Can you work these out from the drawing? Everything is in mm from the part's minimum corner. A direction names the side the tool comes from. Round coordinates to 2 decimals unless told otherwise and drop trailing zeros. Write each loop counter-clockwise with the first axis right and the second up, starting at its lowest first coordinate (ties: lowest second). Pieces come first, ordered by that corner, then holes. Notation, with made-up numbers: (17.25, -27.75) -> (59.25, -27.75) arc R34 ccw to (59.25, 8.25) -> close; hole circle Ø4 at (57.5, 29). An arc over 180 degrees is marked (long way). Answer as CSV lines item,"result". Start each with the question number.
Q1. If I drill on line 1 (Y direction, x = 11.55, z = 17.5); line 2 (Y direction, x = 13.25, z = 17.5); line 3 (X direction, y = 15.5, z = 11.5), over which ranges is the centre line in solid material (lowest first)? Write a range as [from, to].
Q2. For the marked faces 1 and 2, which set-ups out of +Z, -Z, +X, -X, +Y, -Y let a thin tool reach every point of the face, with its end or its side?
Q3. Imagine slicing it at D-D on x = 8. Please give me the cut outline in (y, z).
Q4. If we mould it in two halves opening along Y, with no side actions, what happens to the marked faces 3, 4 and 5? For each: pulls with the +Y half, pulls with the -Y half, needs draft (parallel to the pull), parting line crosses it, or undercut.
Q5. Imagine slicing it at A-A on z = 17.5. Please give me the cut outline in (x, y), and give its area (3 significant figures).
Q6. Will these pins go through, and if not, where does the flat tip stop? pin 1 Ø3 at (y, z) = (46.5, 3.5) entering from +X; pin 2 Ø5 at (y, z) = (8.5, 17.5) entering from +X; pin 3 Ø6.5 at (x, y) = (9.5, 9.5) entering from +Z; pin 4 Ø10 at (x, z) = (8, 10.5) entering from +Y.
Q7. Imagine slicing it at B-B on y = 8. Please give me the cut outline in (x, z), and give its area (3 significant figures).
Q8. Imagine slicing it at C-C on z = 10.5. Please give me the cut outline in (x, y).
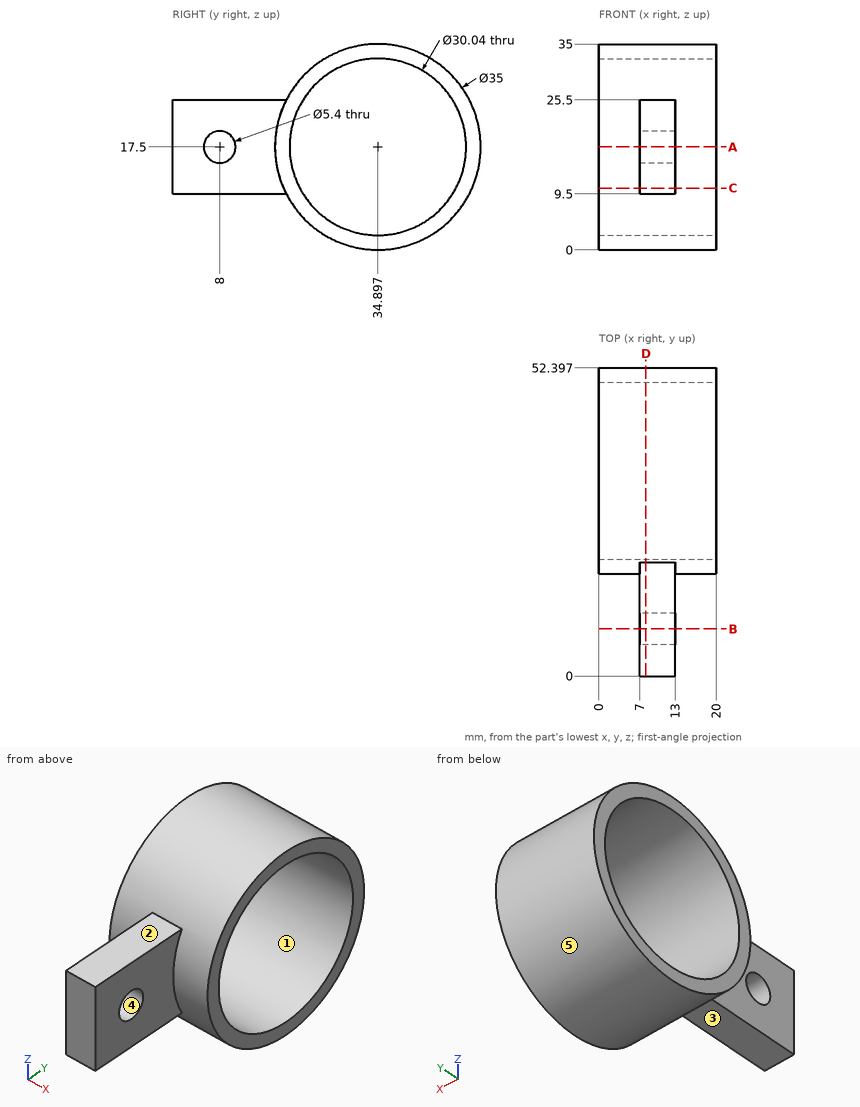
Checks:
1,line 1,"[0, 5.3], [10.7, 19.88], [49.92, 52.4]"
1,line 2,"[17.4, 19.88], [49.92, 52.4]"
1,line 3,"[7, 13]"
2,face 1,"+X, -X"
2,face 2,"+Z, +X, -X, -Y"
3,outline,"(0, 9.5) -> (19.33, 9.5) arc R17.5 ccw (long way) to (19.33, 25.5) -> (0, 25.5) -> close; hole circle Ø5.4 at (8, 17.5); hole circle Ø30.04 at (34.9, 17.5)"
4,face 3,"needs draft"
4,face 4,"undercut"
4,face 5,"parting line crosses it"
5,outline,"(0, 17.4) -> (7, 17.4) -> (7, 10.7) -> (13, 10.7) -> (13, 17.4) -> (20, 17.4) -> (20, 19.88) -> (0, 19.88) -> close; (0, 49.92) -> (20, 49.92) -> (20, 52.4) -> (0, 52.4) -> close; (7, 0) -> (13, 0) -> (13, 5.3) -> (7, 5.3) -> close"
5,area,"171 mm^2"
6,pin 1,"x = 20"
6,pin 2,"x = 13"
6,pin 3,"z = 25.5"
6,pin 4,"y = 52.28"
7,outline,"(7, 9.5) -> (13, 9.5) -> (13, 14.8) -> (7, 14.8) -> close; (7, 20.2) -> (13, 20.2) -> (13, 25.5) -> (7, 25.5) -> close"
7,area,"63.6 mm^2"
8,outline,"(0, 18.86) -> (7, 18.86) -> (7, 0) -> (13, 0) -> (13, 18.86) -> (20, 18.86) -> (20, 21.61) -> (0, 21.61) -> close; (0, 48.19) -> (20, 48.19) -> (20, 50.94) -> (0, 50.94) -> close"
